Design review of the part built by this model. Coordinates are the model's own, in mm. Face numbers are marked on the shaded views. A direction names the side the tool comes from. Coordinates: 2 decimals unless noted, no trailing zeros. Order: outer loops, then holes, each group sorted by start corner. A loop starts at its lowest first (then second) coordinate and runs counter-clockwise, first axis right, second up. Notation, with made-up numbers: (-18.75, -29) - (13.25, -29) arc R7 ccw to (13.25, -25) - close; hole circle Ø7 at (56.5, 41.5). An arc over 180 degrees is marked (long way). Write item = value, one per line. Start each with the question number.
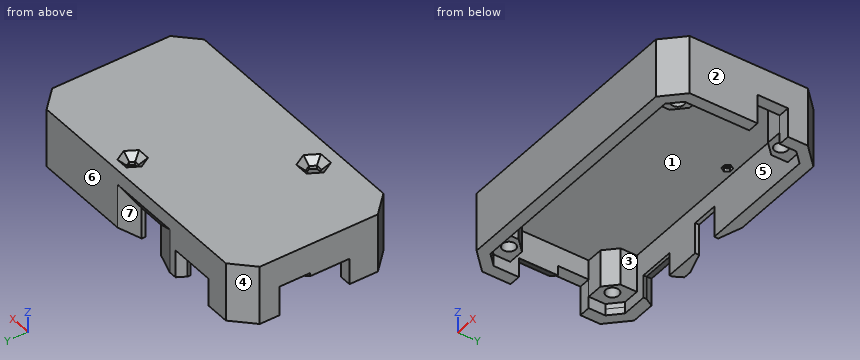
```python
from build123d import *

# Parameters (mm, degrees)
SKETCH_W                      = 88
SKETCH_H                      = 48
PAD_DEPTH                     = 3
SKETCH001_W                   = 88
SKETCH001_H                   = 48
SKETCH001_W_2                 = 81
SKETCH001_H_2                 = 41
PAD001_DEPTH                  = 15
SKETCH002_R                   = 2
PAD002_DEPTH                  = 11.4
SKETCH002_MIRRORED_2_R        = 2
PAD002_MIRRORED_2_DEPTH       = 11.4
SKETCH003_W                   = 9.293619
SKETCH003_H                   = 8.984104
POCKET_DEPTH                  = 5
SKETCH004_W                   = 8.1
SKETCH004_H                   = 9.5
POCKET001_DEPTH               = 5
CHAMFER_ANGLE                 = 18
CHAMFER_SIZE                  = 7
CHAMFER001_ANGLE              = 30
CHAMFER001_SIZE               = 4
SKETCH005_W                   = 11
SKETCH005_H                   = 7
POCKET002_DEPTH               = 5
CHAMFER002_ANGLE              = 60
CHAMFER002_SIZE               = 1.5
PAD003_DEPTH                  = 1.6
PAD003_MIRRORED003_2_DEPTH    = 1.6
POCKET003_DEPTH               = 5
CHAMFER003_SIZE               = 2
POCKET004_DEPTH               = 5
CHAMFER004_SIZE               = 2
SKETCH009_W                   = 12
SKETCH009_H                   = 6
POCKET005_DEPTH               = 5
CHAMFER005_ANGLE              = 60
CHAMFER005_SIZE               = 2
POCKET006_DEPTH               = 221.6870329036
POCKET006_MIRRORED005_2_DEPTH = 221.6870329036
PAD004_DEPTH                  = 2
PAD004_MIRRORED007_2_DEPTH    = 2
BODY_PLACEMENT_ANGLE          = 180


with BuildPart() as part:
    # Sketch → Pad (new body)
    with BuildSketch(Plane.XY):
        Rectangle(SKETCH_W, SKETCH_H)
    extrude(amount=PAD_DEPTH)

    # Sketch001 (on Face6 of Pad) → Pad001 (join)
    with BuildSketch(Plane.XY.offset(3)):
        Rectangle(SKETCH001_W, SKETCH001_H)
        Rectangle(SKETCH001_W_2, SKETCH001_H_2, mode=Mode.SUBTRACT)
    extrude(amount=PAD001_DEPTH)

    # Sketch002 (on Face15 of Pad001) → Pad002 (join)
    with BuildSketch(Plane.XY.offset(3)):
        Polygon((-31.964466094, 15.5), (-31.964466094, 20.5), (-40.5, 20.5), (-40.5, 11.9644660941), (-35.5, 11.9644660941), align=None)
        with Locations((-35.75, 15.75)):
            Circle(SKETCH002_R, mode=Mode.SUBTRACT)
    pad002 = extrude(amount=PAD002_DEPTH)

    # Sketch002 Mirrored 2 → Pad002 Mirrored 2 (add)
    with BuildSketch(Plane(origin=(0, 0, 3), x_dir=(-1, 0, 0), z_dir=(0, 0, -1))):
        Polygon((-31.964466094, 15.5), (-31.964466094, 20.5), (-40.5, 20.5), (-40.5, 11.9644660941), (-35.5, 11.9644660941), align=None)
        with Locations((-35.75, 15.75)):
            Circle(SKETCH002_MIRRORED_2_R, mode=Mode.SUBTRACT)
    pad002_mirrored_2 = extrude(amount=-PAD002_MIRRORED_2_DEPTH)

    # Mirrored001: Pad002, Pad002 Mirrored 2 across Sketch002 H_Axis
    add(pad002.mirror(Plane(origin=(0, 0, 3), x_dir=(0, 0, 1), z_dir=(0, 1, 0))))
    add(pad002_mirrored_2.mirror(Plane(origin=(0, 0, 3), x_dir=(0, 0, 1), z_dir=(0, 1, 0))))

    # Sketch003 (on Face7 of MultiTransform) → Pocket (cut)
    with BuildSketch(Plane(origin=(-44, 0, 0), x_dir=(0, -1, 0), z_dir=(-1, 0, 0))):
        with Locations((7.3011175, 13.507948)):
            Rectangle(SKETCH003_W, SKETCH003_H)
    pocket = extrude(amount=-POCKET_DEPTH, mode=Mode.SUBTRACT)

    # Mirrored002: Pocket across YZ
    add(pocket.mirror(Plane.YZ), mode=Mode.SUBTRACT)

    # Sketch004 (on Face5 of Mirrored002) → Pocket001 (cut)
    with BuildSketch(Plane.XZ.offset(24)):
        with Locations((-3.188932, 13.25)):
            Rectangle(SKETCH004_W, SKETCH004_H)
    extrude(amount=-POCKET001_DEPTH, mode=Mode.SUBTRACT)

    # Chamfer
    chamfer_edges = [part.edges().sort_by_distance(p)[0] for p in [
        (0.861068, -24, 13.25),
        (-7.238932, -24, 13.25),
    ]]
    chamfer_side = part.faces().sort_by_distance((0, -24, 3.892693))[0]
    chamfer(chamfer_edges, length=CHAMFER_SIZE, angle=CHAMFER_ANGLE, reference=chamfer_side)

    # Chamfer001
    chamfer001_edges = [part.edges().sort_by_distance(p)[0] for p in [
        (-3.188932, -24, 8.5),
        (-10.738932, -24, 8.5),
        (4.361068, -24, 8.5),
    ]]
    chamfer001_side = part.faces().sort_by_distance((-29.119466, -24, 17.107307))[0]
    chamfer(chamfer001_edges, length=CHAMFER001_SIZE, angle=CHAMFER001_ANGLE, reference=chamfer001_side)

    # Sketch005 (on Face1 of Chamfer001) → Pocket002 (cut)
    with BuildSketch(Plane.XZ.offset(24)):
        with Locations((-23.6462903219, 14.5)):
            Rectangle(SKETCH005_W, SKETCH005_H)
    extrude(amount=-POCKET002_DEPTH, mode=Mode.SUBTRACT)

    # Chamfer002
    chamfer002_edges = [part.edges().sort_by_distance(p)[0] for p in [
        (-23.64629, -24, 11),
        (-18.14629, -24, 14.5),
        (-29.14629, -24, 14.5),
    ]]
    chamfer002_side = part.faces().sort_by_distance((-10.738932, -24, 3.607307))[0]
    chamfer(chamfer002_edges, length=CHAMFER002_SIZE, angle=CHAMFER002_ANGLE, reference=chamfer002_side)

    # Sketch006 (on Face38 of Chamfer002) → Pad003 (join)
    with BuildSketch(Plane.XY.offset(14.4)):
        Polygon((-40.5, 20.5), (-40.5, 17.0000000001), (-37, 20.5), align=None)
    pad003 = extrude(amount=PAD003_DEPTH)

    # Sketch006 Mirrored003 2 → Pad003 Mirrored003 2 (add)
    with BuildSketch(Plane(origin=(0, 0, 14.4), x_dir=(-1, 0, 0), z_dir=(0, 0, -1))):
        Polygon((-40.5, 20.5), (-40.5, 17.0000000001), (-37, 20.5), align=None)
    pad003_mirrored003_2 = extrude(amount=-PAD003_MIRRORED003_2_DEPTH)

    # Mirrored004: Pad003, Pad003 Mirrored003 2 across Sketch006 H_Axis
    add(pad003.mirror(Plane(origin=(0, 0, 14.4), x_dir=(0, 0, 1), z_dir=(0, 1, 0))))
    add(pad003_mirrored003_2.mirror(Plane(origin=(0, 0, 14.4), x_dir=(0, 0, 1), z_dir=(0, 1, 0))))

    # Sketch007 (on Face27 of MultiTransform001) → Pocket003 (cut)
    with BuildSketch(Plane(origin=(0, 0, 0), x_dir=(1, 0, 0), z_dir=(0, 0, -1))):
        Polygon((-16.267433, -16.921766), (-17.267433, -15.1897151924), (-19.267433, -15.1897151924), (-20.267433, -16.921766), (-19.267433, -18.6538168076), (-17.267433, -18.6538168076), align=None)
    extrude(amount=-POCKET003_DEPTH, mode=Mode.SUBTRACT)

    # Chamfer003
    chamfer003_edges = [part.edges().sort_by_distance(p)[0] for p in [
        (-18.267433, 15.189715, 0),
        (-16.767433, 16.055741, 0),
        (-16.767433, 17.787791, 0),
        (-18.267433, 18.653817, 0),
        (-19.767433, 17.787791, 0),
        (-19.767433, 16.055741, 0),
    ]]
    chamfer(chamfer003_edges, length=CHAMFER003_SIZE)

    # Sketch008 (on Face1 of Chamfer003) → Pocket004 (cut)
    with BuildSketch(Plane(origin=(0, 0, 0), x_dir=(1, 0, 0), z_dir=(0, 0, -1))):
        Polygon((11, 18.25), (10.25, 19.5490381057), (8.75, 19.5490381057), (8, 18.25), (8.75, 16.9509618943), (10.25, 16.9509618943), align=None)
    extrude(amount=-POCKET004_DEPTH, mode=Mode.SUBTRACT)

    # Chamfer004
    chamfer004_edges = [part.edges().sort_by_distance(p)[0] for p in [
        (9.5, -19.549038, 0),
        (8.375, -18.899519, 0),
        (8.375, -17.600481, 0),
        (9.5, -16.950962, 0),
        (10.625, -17.600481, 0),
        (10.625, -18.899519, 0),
    ]]
    chamfer(chamfer004_edges, length=CHAMFER004_SIZE)

    # Sketch009 (on Face25 of Chamfer004) → Pocket005 (cut)
    with BuildSketch(Plane(origin=(-44, 0, 0), x_dir=(0, -1, 0), z_dir=(-1, 0, 0))):
        with Locations((-3.345692, 15)):
            Rectangle(SKETCH009_W, SKETCH009_H)
    extrude(amount=-POCKET005_DEPTH, mode=Mode.SUBTRACT)

    # Chamfer005
    chamfer005_edges = [part.edges().sort_by_distance(p)[0] for p in [
        (-44, 3.345692, 12),
    ]]
    chamfer005_side = part.faces().sort_by_distance((-44, 0.653166, 9.481146))[0]
    chamfer(chamfer005_edges, length=CHAMFER005_SIZE, angle=CHAMFER005_ANGLE, reference=chamfer005_side)

    # Sketch010 (on Face32 of Chamfer005) → Pocket006 (cut, through all)
    with BuildSketch(Plane(origin=(0, 0, 0), x_dir=(1, 0, 0), z_dir=(0, 0, -1))):
        Polygon((38, 24), (44, 24), (44, 18), align=None)
    pocket006 = extrude(amount=-POCKET006_DEPTH, mode=Mode.SUBTRACT)

    # Sketch010 Mirrored005 2 → Pocket006 Mirrored005 2 (cut, through all)
    with BuildSketch(Plane(origin=(0, 0, 0), x_dir=(-1, 0, 0), z_dir=(0, 0, 1))):
        Polygon((38, 24), (44, 24), (44, 18), align=None)
    pocket006_mirrored005_2 = extrude(amount=POCKET006_MIRRORED005_2_DEPTH, mode=Mode.SUBTRACT)

    # Mirrored006: Pocket006, Pocket006 Mirrored005 2 across Sketch010 H_Axis
    add(pocket006.mirror(Plane(origin=(0, 0, 0), x_dir=(0, 0, -1), z_dir=(0, -1, 0))), mode=Mode.SUBTRACT)
    add(pocket006_mirrored005_2.mirror(Plane(origin=(0, 0, 0), x_dir=(0, 0, -1), z_dir=(0, -1, 0))), mode=Mode.SUBTRACT)

    # Sketch011 (on Face32 of MultiTransform002) → Pad004 (join)
    with BuildSketch(Plane.XY.offset(16)):
        Polygon((-40.5, -20.5), (-40.5, -17.0000000001), (-37.0000000001, -20.5), align=None)
    pad004 = extrude(amount=PAD004_DEPTH)

    # Sketch011 Mirrored007 2 → Pad004 Mirrored007 2 (add)
    with BuildSketch(Plane(origin=(0, 0, 16), x_dir=(-1, 0, 0), z_dir=(0, 0, -1))):
        Polygon((-40.5, -20.5), (-40.5, -17.0000000001), (-37.0000000001, -20.5), align=None)
    pad004_mirrored007_2 = extrude(amount=-PAD004_MIRRORED007_2_DEPTH)

    # Mirrored008: Pad004, Pad004 Mirrored007 2 across Sketch011 H_Axis
    add(pad004.mirror(Plane(origin=(0, 0, 16), x_dir=(0, 0, 1), z_dir=(0, 1, 0))))
    add(pad004_mirrored007_2.mirror(Plane(origin=(0, 0, 16), x_dir=(0, 0, 1), z_dir=(0, 1, 0))))


with BuildPart() as part_1:
    # Body placement: moved
    add(part.part.moved(Location((0, 0, 19.4))).rotate(Axis((0, 0, 19.4), (1, 0, 0)), BODY_PLACEMENT_ANGLE))


solid = part_1.part
```
Item 1: For the marked faces 5, 6 and 7, list the 3-axis set-ups (+Z, -Z, +X, -X, +Y, -Y) from which the entire face can be reached by the end or side of a thin tool; tool diameter is ignored.
Item 2: Add section A-A on x = 29. Give the boundary of the cut face in (y, z), plus the area to 3 significant figures.
Item 3: For line 1 (X direction, y = -15.75, z = 8.75); line 2 (Y direction, x = 14, z = 8.25); line 3 (Y direction, x = 35.75, z = 8), list the stretches that pass through material, from the lowest coordinate up.
Item 4: For P1, Ø1.5, axis at x = -39, z = 8.5, coming from the -Y side; P2, Ø1.5, axis at x = -29.5, z = 5.5, coming from the +Y side; P3, Ø1, axis at y = 21, z = 5.5, coming from the +X side; P4, Ø7.5, axis at y = 5.5, z = 8.5, coming from the +X side, all flat-tipped, find the tip position at first contact; note any pin that passes through.
Item 5: Mouldability with a two-part tool opening along Y and no side actions: class the marked faces 1, 2, 3 and 4 as +Y half, -Y half, draft (parallel to the pull), parting line (faces both ways), or undercut.
Item 6: Add section C-C on x = -10. Give the boundary of the cut face in (y, z).
Worked out:
q1.face_5 = -Z
q1.face_6 = +Z, -Z, +X, -X, +Y
q1.face_7 = -Z, +Y
q2.outline = (-24, 1.4) - (-20.5, 1.4) - (-20.5, 16.4) - (20.5, 16.4) - (20.5, 1.4) - (24, 1.4) - (24, 19.4) - (-24, 19.4) - close
q2.area = 249 mm2
q3.line_1 = -44 to -37.75, -33.75 to -31.96, 31.96 to 33.75, 37.75 to 44
q3.line_2 = -24 to -20.5, 20.5 to 24
q3.line_3 = -24 to -17.75, -13.75 to -11.96, 11.96 to 13.75, 17.75 to 24
q4.P1 = -23.75
q4.P2 = 23.31
q4.P3 = 41.5
q4.P4 = 44
q5.face_1 = undercut
q5.face_2 = draft
q5.face_3 = undercut
q5.face_4 = +Y half
q6.outline = (-24, 1.4) - (-20.5, 1.4) - (-20.5, 16.4) - (20.5, 16.4) - (20.5, 1.4) - (22.62, 1.4) - (22.62, 12.51) - (24, 14.9) - (24, 19.4) - (-24, 19.4) - close
